The listing builds one solid part. Answer for the finished solid, in the listing's coordinates (mm). Face numbers are marked on the shaded views. Coordinates: 2 decimals unless noted, no trailing zeros. Write each loop counter-clockwise with the first axis right and the second up, starting at its lowest first coordinate (ties: lowest second). Pieces come first, ordered by that corner, then holes.
from build123d import *

# Parameters (mm, degrees)
BOSS_EXTRU_1_DEPTH           = 5
ESQUISSE3_W                  = 12
ESQUISSE3_H                  = 244.175824176
BOSS_EXTRU_3_DEPTH           = 450
ESQUISSE4_R                  = 2
BOSS_EXTRU_6_DEPTH           = 12
ESQUISSE8_R                  = 5
ENL_V_MAT_EXTRU_2_DEPTH      = 416
BOSS_EXTRU_7_DEPTH           = 110
ENL_V_MAT_EXTRU_6_DEPTH      = 148
ENL_V_MAT_EXTRU_6_DEPTH_BACK = 101
ESQUISSE11_W                 = 303.692307692
ESQUISSE11_H                 = 114.198743449
ENL_V_MAT_EXTRU_8_DEPTH      = 666
ENL_V_MAT_EXTRU_8_DEPTH_BACK = 666
ESQUISSE12_W                 = 140
ESQUISSE12_H                 = 7
ESQUISSE16_W                 = 242.175824176
ESQUISSE16_H                 = 3
BOSS_EXTRU_8_DEPTH           = 15
ESQUISSE17_W                 = 3
ESQUISSE17_H                 = 12
BOSS_EXTRU_11_DEPTH          = 15
ESQUISSE19_W                 = 15
ESQUISSE19_H                 = 12
BOSS_EXTRU_12_DEPTH          = 3
ESQUISSE23_W                 = 110
ESQUISSE23_H                 = 7
BOSS_EXTRU_13_DEPTH          = 12
ESQUISSE24_W                 = 110
ESQUISSE24_H                 = 7
BOSS_EXTRU_14_DEPTH          = 12
ESQUISSE27_W                 = 10
ESQUISSE27_H                 = 338
BOSS_EXTRU_16_DEPTH          = 303.692307692
ESQUISSE28_W                 = 5
ESQUISSE28_H                 = 5
ENL_V_MAT_EXTRU_9_DEPTH      = 15
ESQUISSE29_R                 = 5
ENL_V_MAT_EXTRU_10_DEPTH     = 38
ESQUISSE30_W                 = 303.692307692
ESQUISSE30_H                 = 10
ENL_V_MAT_EXTRU_11_DEPTH     = 340
ESQUISSE31_W                 = 303.692307692
ESQUISSE31_H                 = 10
ENL_V_MAT_EXTRU_12_DEPTH     = 338
BOSS_EXTRU_18_DEPTH          = 10
ESQUISSE34_R                 = 3.644329392
BOSS_EXTRU_19_DEPTH          = 340


with BuildPart() as part:
    # Esquisse1 → Boss.-Extru.1 (new body)
    with BuildSketch(Plane(origin=(0, 0, 0), x_dir=(1, 0, 0), z_dir=(0, 1, 0))):
        Polygon((-125, 166.483516484), (125, 166.483516484), (163.846153846, 122.087912088), (163.846153846, -122.087912088), (125, -166.483516484), (-125, -166.483516484), (-163.846153846, -122.087912088), (-163.846153846, 122.087912088), align=None)
    extrude(amount=BOSS_EXTRU_1_DEPTH)

    # Esquisse3 → Boss.-Extru.3 (add)
    with BuildSketch(Plane.XZ):
        with Locations((-157.846153846, 0)):
            Rectangle(ESQUISSE3_W, ESQUISSE3_H)
        with Locations((157.846153846, 0)):
            Rectangle(ESQUISSE3_W, ESQUISSE3_H)
    extrude(amount=BOSS_EXTRU_3_DEPTH)

    # Esquisse4 → Boss.-Extru.6 (add)
    with BuildSketch(Plane.XZ.offset(450)):
        with Locations(Location((-157.846153846, 67, 0), (0, 0, 90))):
            Circle(ESQUISSE4_R)
        with Locations(Location((-157.846153846, -67, 0), (0, 0, 270))):
            Circle(ESQUISSE4_R)
        with Locations(Location((157.846153846, -67, 0), (0, 0, 90))):
            Circle(ESQUISSE4_R)
        with Locations(Location((157.846153846, 67, 0), (0, 0, 90))):
            Circle(ESQUISSE4_R)
    extrude(amount=BOSS_EXTRU_6_DEPTH)

    # Esquisse8 → Enlèv. mat.-Extru.2 (cut)
    with BuildSketch(Plane.ZY.offset(163.846153846)):
        with Locations((0, -430)):
            Circle(ESQUISSE8_R)
    extrude(amount=-ENL_V_MAT_EXTRU_2_DEPTH, mode=Mode.SUBTRACT)

    # Esquisse10 → Boss.-Extru.7 (add)
    with BuildSketch(Plane(origin=(0, -110, 0), x_dir=(-1, 0, 0), z_dir=(0, -1, 0))):
        Polygon((-163.846153846, 122.087912088), (-125, 166.483516484), (125, 166.483516484), (163.846153846, 122.087912088), (163.846153846, -122.087912088), (125, -166.483516484), (-125, -166.483516484), (-163.846153846, -122.087912088), align=None)
        Polygon((-151.846153846, -122.087912088), (-151.846153846, 122.087912088), (-125.490601914, 152.208542868), (125.490601914, 152.208542868), (151.846153846, 122.087912088), (151.846153846, -122.087912088), (125.490601914, -152.208542868), (-125.490601914, -152.208542868), align=None, mode=Mode.SUBTRACT)
    extrude(amount=-BOSS_EXTRU_7_DEPTH)

    # Esquisse11 → Enlèv. mat.-Extru.6 (cut, two sides: drawn at the far end of the back side and taken through both)
    with BuildSketch(Plane(origin=(0, 0, 152.208542868), x_dir=(-1, 0, 0), z_dir=(0, 0, -1)).offset(-ENL_V_MAT_EXTRU_6_DEPTH_BACK)):
        with Locations((0, -62.099371725)):
            Rectangle(ESQUISSE11_W, ESQUISSE11_H)
    extrude(amount=ENL_V_MAT_EXTRU_6_DEPTH + ENL_V_MAT_EXTRU_6_DEPTH_BACK, mode=Mode.SUBTRACT)

    # Esquisse12 → Enlèv. mat.-Extru.8 (cut, two sides: drawn at the far end of the back side and taken through both)
    with BuildSketch(Plane.ZY.offset(-151.846153846).offset(-ENL_V_MAT_EXTRU_8_DEPTH_BACK)):
        with Locations((0, -332.164926547)):
            Rectangle(ESQUISSE12_W, ESQUISSE12_H)
    extrude(amount=ENL_V_MAT_EXTRU_8_DEPTH + ENL_V_MAT_EXTRU_8_DEPTH_BACK, mode=Mode.SUBTRACT)

    # Esquisse16 → Boss.-Extru.8 (add)
    with BuildSketch(Plane(origin=(-151.846153846, 0, 0), x_dir=(0, 0, -1), z_dir=(1, 0, 0))):
        with Locations((1, -108.5)):
            Rectangle(ESQUISSE16_W, ESQUISSE16_H)
        with Locations((1, -99.5)):
            Rectangle(ESQUISSE16_W, ESQUISSE16_H)
    boss_extru_8 = extrude(amount=BOSS_EXTRU_8_DEPTH)

    # Esquisse17 → Boss.-Extru.11 (add)
    with BuildSketch(Plane(origin=(-136.846153846, 0, 0), x_dir=(0, 0, -1), z_dir=(1, 0, 0))):
        with Locations((120.587912088, -104)):
            Rectangle(ESQUISSE17_W, ESQUISSE17_H)
    extrude(amount=-BOSS_EXTRU_11_DEPTH)

    # Symétrie2: Boss.-Extru.8 across plane
    add(boss_extru_8.mirror(Plane(origin=(0, 0, 0), x_dir=(0, 0, 1), z_dir=(1, 0, 0))))

    # Esquisse19 → Boss.-Extru.12 (add)
    with BuildSketch(Plane(origin=(0, 0, -122.087912088), x_dir=(-1, 0, 0), z_dir=(0, 0, -1))):
        with Locations((-144.346153846, -104)):
            Rectangle(ESQUISSE19_W, ESQUISSE19_H)
    extrude(amount=-BOSS_EXTRU_12_DEPTH)

    # Esquisse23 → Boss.-Extru.13 (add)
    with BuildSketch(Plane(origin=(-151.846153846, 0, 0), x_dir=(0, 0, -1), z_dir=(1, 0, 0))):
        with Locations((0, -332.164926547)):
            Rectangle(ESQUISSE23_W, ESQUISSE23_H)
    extrude(amount=-BOSS_EXTRU_13_DEPTH)

    # Esquisse24 → Boss.-Extru.14 (add)
    with BuildSketch(Plane(origin=(163.846153846, 0, 0), x_dir=(0, 0, -1), z_dir=(1, 0, 0))):
        with Locations((0, -332.164926547)):
            Rectangle(ESQUISSE24_W, ESQUISSE24_H)
    extrude(amount=-BOSS_EXTRU_14_DEPTH)

    # Esquisse27 → Boss.-Extru.16 (add)
    with BuildSketch(Plane.ZY.offset(-151.846153846)):
        with Locations((-82.501488258, -281)):
            Rectangle(ESQUISSE27_W, ESQUISSE27_H)
    boss_extru_16 = extrude(amount=BOSS_EXTRU_16_DEPTH)

    # Symétrie4: Boss.-Extru.16 across plane
    add(boss_extru_16.mirror(Plane.XY))

    # Esquisse28 → Enlèv. mat.-Extru.9 (cut)
    with BuildSketch(Plane(origin=(0, 5, 0), x_dir=(1, 0, 0), z_dir=(0, 1, 0))):
        with Locations((-115.95070095, 4.416314077)):
            Rectangle(ESQUISSE28_W, ESQUISSE28_H)
    extrude(amount=-ENL_V_MAT_EXTRU_9_DEPTH, mode=Mode.SUBTRACT)

    # Esquisse29 → Enlèv. mat.-Extru.10 (cut)
    with BuildSketch(Plane(origin=(163.846153846, 0, 0), x_dir=(0, 0, -1), z_dir=(1, 0, 0))):
        with Locations((0, -382.55)):
            Circle(ESQUISSE29_R)
    extrude(amount=-ENL_V_MAT_EXTRU_10_DEPTH, mode=Mode.SUBTRACT)

    # Esquisse30 → Enlèv. mat.-Extru.11 (cut)
    with BuildSketch(Plane.XZ.offset(450)):
        with Locations((0, 82.501488258)):
            Rectangle(ESQUISSE30_W, ESQUISSE30_H)
    extrude(amount=-ENL_V_MAT_EXTRU_11_DEPTH, mode=Mode.SUBTRACT)

    # Esquisse31 → Enlèv. mat.-Extru.12 (cut)
    with BuildSketch(Plane.XZ.offset(450)):
        with Locations((0, -82.501488258)):
            Rectangle(ESQUISSE31_W, ESQUISSE31_H)
    extrude(amount=-ENL_V_MAT_EXTRU_12_DEPTH, mode=Mode.SUBTRACT)

    # Esquisse33 → Boss.-Extru.18 (add)
    with BuildSketch(Plane(origin=(0, -110, 0), x_dir=(-1, 0, 0), z_dir=(0, -1, 0))):
        Polygon((-21.957412763, 185.323052507), (21.957412763, 185.323052507), (34.400295625, 166.483516484), (-34.400295625, 166.483516484), align=None)
    extrude(amount=-BOSS_EXTRU_18_DEPTH)

    # Esquisse34 → Boss.-Extru.19 (add)
    with BuildSketch(Plane.XZ.offset(110)):
        with Locations(Location((0, -177.983018986, 0), (0, 0, 90))):
            Circle(ESQUISSE34_R)
    extrude(amount=BOSS_EXTRU_19_DEPTH)


solid = part.part
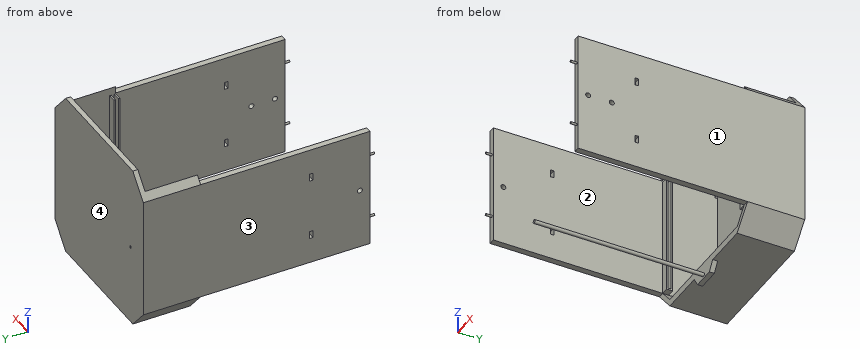
Q1. Given pin 1 (3 mm diameter, centred on x = -5.5, y = -337, fed in from -Z); pin 2 (1 mm diameter, centred on y = -66, z = 124.5, fed in from +X); pin 3 (3.5 mm diameter, centred on x = -157, z = -54.5, fed in from -Y); pin 4 (1.5 mm diameter, centred on x = -14.5, z = 12, fed in from -Y), each flat-ended and moving along its own axis, determine where each tip first touches the part or whether it passes through.
Answers below:
pin 1: passes through
pin 2: stops at x = 162.17
pin 3: stops at y = -450
pin 4: stops at y = 0
Q2. The part is cut by section D-D, the plane y = -52.5. Write down the section's boundary in (x, z).
Answers below:
outline: (-163.85, -122.09) - (-125, -166.48) - (125, -166.48) - (163.85, -122.09) - (163.85, 122.09) - (151.85, 135.8) - (151.85, -122.09) - (125.49, -152.21) - (-125.49, -152.21) - (-151.85, -122.09) - (-151.85, 135.8) - (-163.85, 122.09) - close
Q3. Determine the mould class of the marked faces 1, 2, 3 and 4 for opening direction X: released by +X, released by -X, zero draft, split by the parting line, or undercut.
Answers below:
face 1: released by +X
face 2: undercut
face 3: released by -X
face 4: zero draft
Q4. The part is cut by section C-C, the plane z = 85.5. Write down the section's boundary in (x, y), then the cut area to 3 significant figures.
Answers below:
outline: (-163.85, -450) - (-151.85, -450) - (-151.85, -110) - (-136.85, -110) - (-136.85, -107) - (-151.85, -107) - (-151.85, -101) - (-136.85, -101) - (-136.85, -98) - (-151.85, -98) - (-151.85, 0) - (151.85, 0) - (151.85, -98) - (136.85, -98) - (136.85, -101) - (151.85, -101) - (151.85, -107) - (136.85, -107) - (136.85, -110) - (151.85, -110) - (151.85, -450) - (163.85, -450) - (163.85, 5) - (-163.85, 5) - close
area: 12,600 mm2
Q5. The part is cut by section B-B, the plane x = -11.5. Write down the section's boundary in (y, z), then the cut area to 3 significant figures.
Answers below:
outline: (-110, -185.32) - (-100, -185.32) - (-100, -166.48) - (5, -166.48) - (5, 166.48) - (-5, 166.48) - (-5, 152.21) - (0, 152.21) - (0, -152.21) - (-110, -152.21) - close
area: 3,490 mm2
Q6. Find the intervals of material crossed by probe 1 along Y at (x, z) = (160.5, 0); probe 2 along X at (y, z) = (-293, -93); probe 3 along Y at (x, z) = (-158.5, 0), in increasing order.
Answers below:
probe 1: y = -450 to -435, -425 to -387.55, -377.55 to 5
probe 2: x = -163.85 to -151.85, 151.85 to 163.85
probe 3: y = -450 to -435, -425 to 5
Q7. The part is cut by section A-A, the plane y = -344.5. Write down the section's boundary in (x, z), then the cut area to 3 significant figures.
Answers below:
outline: (-163.85, -122.09) - (-151.85, -122.09) - (-151.85, 122.09) - (-163.85, 122.09) - close; circle Ø7.29 at (0, -177.98); (151.85, -122.09) - (163.85, -122.09) - (163.85, 122.09) - (151.85, 122.09) - close
area: 5,900 mm2
